Source: three-view drawing plus pictorial views. Frame: mm from the lowest corner of the part. Give positions to 0.01 mm unless a question says otherwise; leave off trailing zeros. Loops run counter-clockwise (first coordinate to the right, second up) from the corner with the lowest first, then second, coordinate; pieces in that order, holes last.
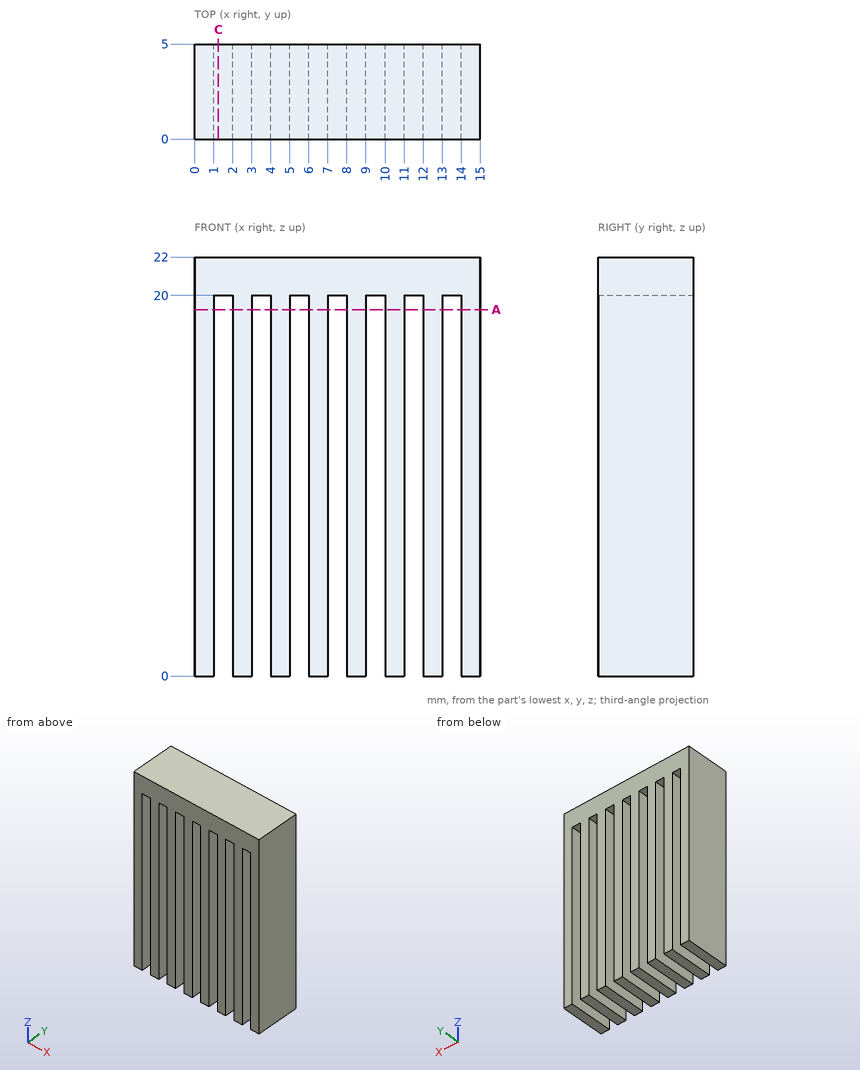
(1) Cut plane C-C (x = 1.25). Return the cut outline in (y, z), and give its area (3 significant figures).
Values follow:
outline: (0, 20) - (5, 20) - (5, 22) - (0, 22) - close
area: 10.0 mm2
(2) Pin query (flat end, axial travel): pin 1 Ø0.8 at (x, y) = (7.5, 2) entering from -Z. Return the tip coordinate at first contact, or that it passes through.
Values follow:
pin 1: stops at z = 20
(3) Ray query, probe 1 along Z at (x, y) = (3.75, 4.25). Return the intervals inside material, ascending.
Values follow:
probe 1: z = 20 to 22
(4) Cut plane A-A (z = 19.25). Count the separate pieces of the cut face and the enclosed holes in it, and give its area (3 significant figures).
Values follow:
separate pieces: 8
enclosed holes: 0
area: 40.0 mm2
